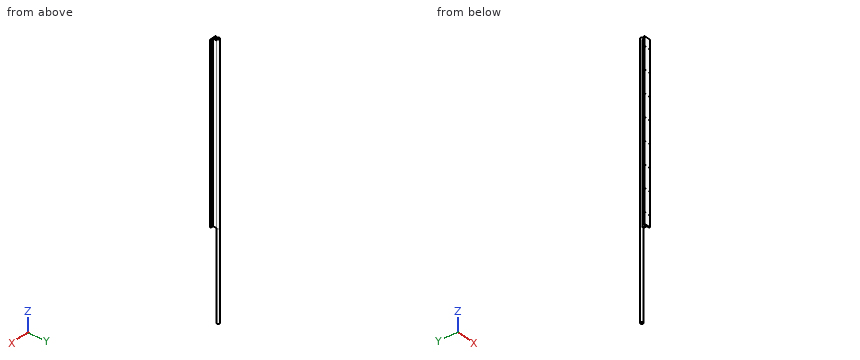
from build123d import *
from build123d.topology import SkipClean

# Parameters (mm, degrees)
EXTRUDE1_DEPTH         = 1219.2
F_10_CLEARANCE_HOLE1_D = 5.6134
LPATTERN3_COUNT        = 8
LPATTERN3_PITCH        = 152.4
SKETCH4_OUTSIDE_W      = 290.638
SKETCH4_OUTSIDE_H      = 293.813
SKETCH4_OUTSIDE_R      = 9.525
CUT_EXTRUDE1_DEPTH     = 12.7
EXTRUDE2_START         = 609.6
SKETCH5_R              = 9.525
EXTRUDE2_DEPTH         = 609.6


with BuildPart() as part:
    # Sketch1 → Extrude1 (new body)
    with BuildSketch(Plane.XY):
        with BuildLine():
            Line((-22.225, -38.1), (22.225, -38.1))
            Line((22.225, -38.1), (22.225, -31.75))
            Line((22.225, -31.75), (4.7625, -31.75))
            Line((4.7625, -31.75), (4.7625, -8.248891971))
            ThreePointArc((4.7625, -8.248891971), (0, 9.525), (-4.7625, -8.248891971))
            Line((-4.7625, -8.248891971), (-4.7625, -31.75))
            Line((-4.7625, -31.75), (-22.225, -31.75))
            Line((-22.225, -31.75), (-22.225, -38.1))
        make_face()
    extrude(amount=EXTRUDE1_DEPTH)

    # #10 Clearance Hole1 (through all)
    with Locations(Plane.XZ.offset(38.1)):
        with Locations((-15.875, 76.2), (15.875, 76.2)):
            f_10_clearance_hole1 = Hole(F_10_CLEARANCE_HOLE1_D / 2)

    # LPattern3: #10 Clearance Hole1 ×8
    with Locations(*[(0, 0, i * LPATTERN3_PITCH) for i in range(1, LPATTERN3_COUNT)]):
        add(f_10_clearance_hole1, mode=Mode.SUBTRACT)

    # Sketch4 outside → Cut-Extrude1 (cut)
    with BuildSketch(Plane.XY.offset(1219.2)):
        with Locations((0, -14.2875)):
            Rectangle(SKETCH4_OUTSIDE_W, SKETCH4_OUTSIDE_H)
        with Locations(Location((0, 0, 0), (0, 0, 240))):
            Circle(SKETCH4_OUTSIDE_R, mode=Mode.SUBTRACT)
    extrude(amount=-CUT_EXTRUDE1_DEPTH, mode=Mode.SUBTRACT)

    # Sketch5 → Extrude2 (add)
    with SkipClean():  # the faces are left unmerged after this step: merging them gives an invalid solid
        with BuildSketch(Plane(origin=(0, 0, 0), x_dir=(-1, 0, 0), z_dir=(0, 0, -1)).offset(EXTRUDE2_START)):
            Circle(SKETCH5_R)
        extrude(amount=-EXTRUDE2_DEPTH)


solid = part.part
Can you work these out from the model? Positions are in its coordinate system, mm. Give positions to 0.01 mm unless a question says otherwise; leave off trailing zeros. Loops run counter-clockwise (first coordinate to the right, second up) from the corner with the lowest first, then second, coordinate; pieces in that order, holes last. Notation, with made-up numbers: (19.25, 2.5) -> (63.25, 2.5) arc R20 cw to (63.25, 25.5) -> close; hole circle Ø9 at (81.25, -39.5). An arc over 180 degrees is marked (long way). Use one line per item in the form item = value.
1) Will these pins go through, and if not, where does the flat tip stop? pin 1 (2 mm diameter, centred on y = -15.5, z = 719, fed in from -X); pin 2 (19 mm diameter, centred on x = -11.5, z = 754, fed in from +Y); pin 3 (1 mm diameter, centred on y = -9, z = 909, fed in from +X); pin 4 (5 mm diameter, centred on x = -15.875, z = 990.6, fed in from -Y).
Answers:
pin_1 = -4.76
pin_2 = 9.31
pin_3 = 4.76
pin_4 = through
2) If we section it at C-C (z = -328.5): Please give me the cut outline in (x, y) (3 decimals), plus the area to 3 significant figures.
Answers:
outline = circle Ø19.05 at (0, 0)
area = 285 mm²
3) I need wall thicknesses on line 1 along X through (y, z) = (-36, 228) (3 decimals); line 2 along X through (y, z) = (-33.75, 838.2) (3 decimals); line 3 along Y through (x, z) = (20.5, 135). Which ranges of each line are inside material? Lowest first, please.
Answers:
line_1 = -22.225 to -18.617, -13.133 to 13.133, 18.617 to 22.225
line_2 = -22.225 to -18.682, -13.068 to 13.068, 18.682 to 22.225
line_3 = -38.1 to -31.75
4) If we section it at B-B (y = 0): Please give me the cut outline in (x, z) (3 decimals), plus the area to 3 significant figures.
Answers:
outline = (-9.525, -609.6) -> (9.525, -609.6) -> (9.525, 1219.2) -> (-9.525, 1219.2) -> close
area = 34,800 mm²
